Here's how the part is built. I have some questions about the finished solid (model axes, mm). A direction names the side the tool comes from. Coordinates: 2 decimals unless noted, no trailing zeros. Write each loop counter-clockwise with the first axis right and the second up, starting at its lowest first coordinate (ties: lowest second). Pieces come first, ordered by that corner, then holes. Notation, with made-up numbers: M 32.25,-30.5 L 36.25,-30.5 A17 ccw 36.25,-7.5 Z; hole C 41.25,-39 d11. An arc over 180 degrees is marked long. Use a Markdown table: item, result.
Autodesk Inventor part; units mm, degrees
ref_plane "YZ Plane" through (0, 0, 0) normal (1, 0, 0) x (0, 1, 0)
ref_plane "XZ Plane" through (0, 0, 0) normal (0, 1, 0) x (-1, 0, 0)
ref_plane "XY Plane" through (0, 0, 0) normal (0, 0, 1) x (1, 0, 0)
sketch "Sketch1" plane through (0, 0, 0) normal (0, 1, 0) x (-1, 0, 0)
  line L0 (0, 0) -> (50, 0)
  line L1 (50, 0) -> (50, 50)
  line L2 (50, 50) -> (0, 50)
  line L3 (0, 50) -> (0, 0)
  circle A0 centre (12, 43) radius 2.375
  circle A1 centre (43, 43) radius 2.375
  circle A2 centre (43, 12) radius 2.375
  circle A3 centre (12, 12) radius 2.375
  circle A4 centre (27.5, 27.5) radius 12.5
  line L4 (43, 12) -> (27.5, 27.5) construction
  line L5 (27.5, 27.5) -> (12, 43) construction
  dimension "d0" = 50
  dimension "d1" = 50
  dimension "d2" = 4.75
  dimension "d3" = 31
  dimension "d4" = 31
  dimension "d5" = 7
  dimension "d6" = 7
  dimension "d7" = 25
extrude "Extrusion1" add sketch "Sketch1" along normal blind 6
sketch "Sketch2" plane through (0, 6, 0) normal (0, 1, 0) x (1, 0, 0)
  line L0 (0, 0) -> (-50, 0)
  line L1 (0, -50) -> (0, 0)
  line L2 (-50, 0) -> (0, 0)
  line L3 (0, -50) -> (-6, -50)
  line L4 (-6, -6) -> (-50, -6)
  line L5 (-6, -6) -> (-6, -50)
  line L6 (-50, -6) -> (-50, 0)
  line L7 (0, -50) -> (-6, -50)
  line L8 (0, 0) -> (0, -50)
  dimension "d10" = 6
extrude "Extrusion2" add sketch "Sketch2" along normal blind 15
sketch "Sketch3" plane through (-6, 6, 6) normal (-1, 0, 0) x (0, 0, 1)
  line L0 (0, 0) -> (0, 15)
  circle A0 centre (6, 7.5) radius 2.5
  circle A1 centre (37, 7.5) radius 2.5
  line L1 (0, 7.5) -> (6, 7.5) construction
  line L2 (6, 7.5) -> (37, 7.5) construction
  point P0 (-6, -6)
  dimension "d13" = 6
  dimension "d14" = 31
  dimension "d15" = 5
extrude "Extrusion3" cut sketch "Sketch3" against normal blind 15
equation "\"d1\" = d0"
equation "\"d4\" = d3"
equation "\"d6\" = d5"
properties part number "motorMount"
1. Suppose I cut it at C-C on z = 27.5. Write out the boundary of the cut face in (x, y), and give its area (3 significant figures).
Answers follow:
| item | result |
|---|---|
| outline | M -50,0 L -40,0 L -40,6 L -50,6 Z; M -15,0 L 0,0 L 0,21 L -6,21 L -6,6 L -15,6 Z |
| area | 240 mm2 |
2. Which directions (+Z, -Z, +X, -X, +Y, -Y) give clear straight access to the entire face, cutting with the end or side of a thin tool? Please do faces 4 (the face through (-37, 6, 19)), 5 (the face through (-16, 21, 5)).
Answers follow:
| item | result |
|---|---|
| face 4 | +Z, -X, +Y |
| face 5 | +Z, -Z, +X, -X, +Y |
3. We'd pull the mould along Y, two halves only. Please class faces 1 (the face through (-3.04, 12.54, 45.31)), 2 (the face through (-25, 0, 14)), 3 (the face through (-6, 13, 28)): +Y half, -Y half, draft (parallel to the pull), parting line (faces both ways), or undercut.
Answers follow:
| item | result |
|---|---|
| face 1 | undercut |
| face 2 | -Y half |
| face 3 | draft |
4. I need wall thicknesses on probe 1 along Z at (x, y) = (-27.5, 1.2); probe 2 along Z at (x, y) = (-12, 2.75) (3 decimals); probe 3 along Y at (x, z) = (-3.4, 43). Which ranges of each line are inside material? Lowest first, please.
Answers follow:
| item | result |
|---|---|
| probe 1 | z = 0 to 15, 40 to 50 |
| probe 2 | z = 0 to 9.625, 14.375 to 40.625, 45.375 to 50 |
| probe 3 | y = 0 to 11, 16 to 21 |
5. Suppose I cut it at A-A on y = 13.5. Write out the boundary of the cut face in (x, z), and give its area (3 significant figures).
Answers follow:
| item | result |
|---|---|
| outline | M -50,0 L 0,0 L 0,9.5 L -6,9.5 L -6,6 L -50,6 Z; M -6,14.5 L 0,14.5 L 0,40.5 L -6,40.5 Z; M -6,45.5 L 0,45.5 L 0,50 L -6,50 Z |
| area | 504 mm2 |
6. Will these pins go through, and if not, where does the flat tip stop? pin 1 Ø12 at (x, z) = (-33, 43) entering from +Y; pin 2 Ø8 at (y, z) = (13.5, 43) entering from -X; pin 3 Ø3 at (x, y) = (-26.5, 9) entering from +Z; pin 4 Ø3 at (x, z) = (-12, 12) entering from +Y.
Answers follow:
| item | result |
|---|---|
| pin 1 | stops at y = 6 |
| pin 2 | stops at x = -6 |
| pin 3 | stops at z = 6 |
| pin 4 | passes through |
7. Suppose I cut it at B-B on x = -27.5. Write out the boundary of the cut face in (y, z).
Answers follow:
| item | result |
|---|---|
| outline | M 0,0 L 21,0 L 21,6 L 6,6 L 6,15 L 0,15 Z; M 0,40 L 6,40 L 6,50 L 0,50 Z |
8. Suppose I cut it at D-D on x = -43. Write out the boundary of the cut face in (y, z) (3 decimals), and give its area (3 significant figures).
Answers follow:
| item | result |
|---|---|
| outline | M 0,0 L 21,0 L 21,6 L 6,6 L 6,9.625 L 0,9.625 Z; M 0,14.375 L 6,14.375 L 6,40.625 L 0,40.625 Z; M 0,45.375 L 6,45.375 L 6,50 L 0,50 Z |
| area | 333 mm2 |
